Check sheet for the modelled part. Datum: model origin and axes. Units: mm. A direction names the side the tool comes from. Give positions to 0.01 mm unless a question says otherwise; leave off trailing zeros. Write each loop counter-clockwise with the first axis right and the second up, starting at its lowest first coordinate (ties: lowest second). Pieces come first, ordered by that corner, then holes. Notation, with made-up numbers: (-10.5, -28) -> (35.5, -28) arc R17 cw to (35.5, -20) -> close; hole circle Ø3 at (53, 28.5). An arc over 180 degrees is marked (long way). Use a Markdown table: item, result. Add a question column.
1. Gauge pin test, flat end, axial feed: P1, Ø0.5, axis at x = -44.5, y = -16, coming from the -Z side. Record the tip position at first contact, or that the pin passes through.
2. Cross-section at B-B (x = -66). Enter the section's corners in (y, z) (3 decimals).
3. Set-up check for faces 4 (the flat face through (-25, -13, 0.178)), 5 (the flat face through (-82.55, -13, 1)), 6 (the flat face through (-76.981, -13.443, -0.996)): record each of +Z, -Z, +X, -X, +Y, -Y from which the full face is reachable in a straight line by a thin tool's end or side.
4. Release check for a two-part mould opening along Z. For faces 1 (the flat face through (-37, -19.685, 2)), 2 (the flat face through (-38, -13, 0.178)), 3 (the flat face through (-77.05, -13.44, -3.29)) record: released by +Z, released by -Z, zero draft, split by the parting line, or undercut.
5. Cross-section at A-A (z = -1). Enter the section's corners in (x, y) (3 decimals), then the cut area to 3 significant figures.
6. Scan lines: probe 1 along X at (y, z) = (-12.5, -3.5); probe 2 along Z at (x, y) = (-2, -17); probe 3 along X at (y, z) = (-18.25, -4). Record each from-to range of solid material in increasing order. Write a range as [from, to].
Solid Edge part; units mm, degrees
sketch "Sketch1" plane through (0, 0, 0) normal (0, 0, 1) x (1, 0, 0)
  line L0 (6.35, -7.0244) -> (6.35, -19.685)
  line L1 (6.35, -19.685) -> (-82.55, -19.685)
  line L2 (-82.55, -19.685) -> (-82.55, -7.0244)
  line L3 (-82.55, -7.0244) -> (6.35, -7.0244)
extrude "Protrusion1" add sketch "Sketch1" against normal up to vertex (4.4079 mm away)
sketch "Sketch2" plane through (0, 0, 0) normal (0, 0, 1) x (1, 0, 0)
  line L0 (6.35, -19.685) -> (-82.55, -19.685)
  line L1 (-82.55, -19.685) -> (-82.55, -7.0244)
  line L2 (-82.55, -7.0244) -> (6.35, -7.0244)
  line L3 (6.35, -7.0244) -> (6.35, -19.685)
extrude "Protrusion2" add sketch "Sketch2" along normal blind 6.35
sketch "Sketch3" plane through (-38.1, -19.685, 0.971) normal (0, -1, 0) x (1, 0, 0)
  line L0 (38.2778, -11.6851) -> (38.2778, -5.4266)
  line L1 (38.2778, -5.4266) -> (39.5778, -3.175)
  line L2 (39.5778, -3.175) -> (38.2027, -0.7932)
  line L3 (38.2027, -0.7932) -> (34.0828, -0.7932)
  line L4 (34.0828, -0.7932) -> (-38.2027, -0.7932)
  line L5 (-38.2027, -0.7932) -> (-39.5778, -3.175)
  line L6 (-39.5778, -3.175) -> (-38.2778, -5.4266)
  line L7 (-38.2778, -5.4266) -> (-38.2778, -11.6851)
  line L8 (-38.2778, -11.6851) -> (38.2778, -11.6851)
extrude "Cutout1" cut sketch "Sketch3" against normal through all
sketch "Sketch4" plane through (-38.1, -19.685, 0.971) normal (0, -1, 0) x (1, 0, 0)
  line L0 (34.0828, -1.6488) -> (34.0828, -0.7932)
  line L1 (34.0828, -0.7932) -> (34.0828, -0.1248)
  line L2 (33.2272, -0.1248) -> (34.0828, -0.1248)
  line L3 (33.2272, -0.7932) -> (33.2272, -0.1248)
  line L4 (33.2272, -0.7932) -> (33.2272, -1.6488)
  line L5 (33.2272, -1.6488) -> (34.0828, -1.6488)
  line L6 (32.8128, -1.6488) -> (32.8128, -0.7932)
  line L7 (32.8128, -0.7932) -> (32.8128, -0.1248)
  line L8 (31.9572, -0.1248) -> (32.8128, -0.1248)
  line L9 (31.9572, -0.7932) -> (31.9572, -0.1248)
  line L10 (31.9572, -0.7932) -> (31.9572, -1.6488)
  line L11 (31.9572, -1.6488) -> (32.8128, -1.6488)
  line L12 (31.5428, -1.6488) -> (30.6872, -1.6488)
  line L13 (30.6872, -1.6488) -> (30.6872, -0.7932)
  line L14 (30.6872, -0.7932) -> (30.6872, -0.1248)
  line L15 (30.6872, -0.1248) -> (31.5428, -0.1248)
  line L16 (31.5428, -0.7932) -> (31.5428, -0.1248)
  line L17 (31.5428, -0.7932) -> (31.5428, -1.6488)
  line L18 (30.2728, -1.6488) -> (29.4172, -1.6488)
  line L19 (29.4172, -1.6488) -> (29.4172, -0.7932)
  line L20 (29.4172, -0.1248) -> (29.4172, -0.7932)
  line L21 (29.4172, -0.1248) -> (30.2728, -0.1248)
  line L22 (30.2728, -0.7932) -> (30.2728, -0.1248)
  line L23 (30.2728, -0.7932) -> (30.2728, -1.6488)
extrude "Cutout2" cut sketch "Sketch4" against normal through all
pattern_linear "Pattern1" count 5 spacing 12.7 along (-1, 0, 0) of "Cutout2"
Worked answers:
| question | item | result |
|---|---|---|
| 1 | P1 | stops at z = 0.18 |
| 2 | outline | (-19.685, 0.178) -> (-7.024, 0.178) -> (-7.024, 6.35) -> (-19.685, 6.35) -> close |
| 3 | face 4 | -Z, +Y, -Y |
| 3 | face 5 | +Z, -Z, -X, +Y, -Y |
| 3 | face 6 | +Y, -Y |
| 4 | face 1 | zero draft |
| 4 | face 2 | released by -Z |
| 4 | face 3 | undercut |
| 5 | outline | (-82.55, -19.685) -> (-76.983, -19.685) -> (-76.983, -7.024) -> (-82.55, -7.024) -> close; (0.783, -19.685) -> (6.35, -19.685) -> (6.35, -7.024) -> (0.783, -7.024) -> close |
| 5 | area | 141 mm² |
| 6 | probe 1 | x = [-82.55, -76.93], [0.73, 6.35] |
| 6 | probe 2 | z = [0.18, 6.35] |
| 6 | probe 3 | x = [-82.55, -76.64], [0.44, 6.35] |
